Can you work these out from the model? Positions are in its coordinate system, mm. Face numbers are marked on the shaded views. A direction names the side the tool comes from. Coordinates: 2 decimals unless noted, no trailing zeros. Order: outer loops, then holes, each group sorted by start corner. A loop starts at its lowest first (then second) coordinate and runs counter-clockwise, first axis right, second up. Notation, with made-up numbers: (27, 82) -> (84, 82) arc R19 cw to (84, 87) -> close; hole circle Ø5 at (64, 70.25). An arc over 180 degrees is marked (long way). Return JSON: item names as keys, results as strings. Group by question number.
1) If we section it at A-A, the plane x = -5: Please give me the cut outline in (y, z), then the cut area to 3 significant figures.
2) For pin 1 (21.5 mm diameter, centred on x = -15.5, y = 22, fed in from -Z); pin 2 (4 mm diameter, centred on y = 12, z = 23, fed in from +X); pin 3 (4 mm diameter, centred on y = 12, z = 47, fed in from -X); pin 4 (12 mm diameter, centred on y = 44.5, z = 20.5, fed in from +X), each with a flat end and sliding along its axis, tell me the tip position at first contact or that it passes through.
3) If we section it at C-C, the plane y = 36: Please give me the cut outline in (x, z), then the cut area to 3 significant figures.
4) If we section it at D-D, the plane z = 47: Please give me the cut outline in (x, y).
5) If I drill on probe 1 along Y at (x, z) = (-44.15, 55); probe 2 along X at (y, z) = (58, 7); probe 3 along Z at (x, y) = (-28.5, 36), over which ranges is the centre line in solid material (lowest first)? Write a range as from..to.
6) For the marked faces 1 and 2, which set-ups out of +Z, -Z, +X, -X, +Y, -Y let a thin tool reach every point of the face, with its end or its side?
7) If we section it at B-B, the plane z = 56: Please give me the cut outline in (x, y), then the cut area to 3 significant figures.
8) Thinking about a two-plate mould opening in Z: for the marked faces 3, 4, 5 and 6, which applies, +Z half, -Z half, draft (parallel to the pull), parting line (faces both ways), or undercut?
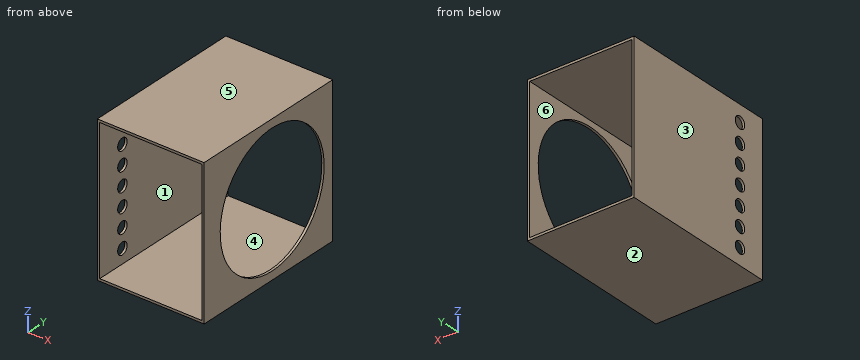
Autodesk Inventor part; units mm, degrees
ref_plane "YZ Plane" through (0, 0, 0) normal (1, 0, 0) x (0, 1, 0)
ref_plane "XZ Plane" through (0, 0, 0) normal (0, 1, 0) x (-1, 0, 0)
ref_plane "XY Plane" through (0, 0, 0) normal (0, 0, 1) x (1, 0, 0)
sketch "Boceto1" plane through (0, 0, 0) normal (0, 1, 0) x (-1, 0, 0)
  line L0 (0, 0) -> (45, 0)
  line L1 (45, 0) -> (45, 62)
  line L2 (45, 62) -> (0, 62)
  line L3 (0, 62) -> (0, 0)
  line L4 (44, 61) -> (1, 61)
  line L5 (1, 61) -> (1, 1)
  line L6 (1, 1) -> (44, 1)
  line L7 (44, 1) -> (44, 61)
  point P0 (22.5, 62)
  dimension "d0" = 1
  dimension "d1" = 1
  dimension "d2" = 1
  dimension "d3" = 1
  dimension "d4" = 43
  dimension "d5" = 60
extrude "Extrusión1" add sketch "Boceto1" along normal blind 68
sketch "Boceto2" plane through (0, 0, 62) normal (1, 0, 0) x (0, 0, -1)
  line L0 (0, 0) -> (62, 0)
  line L1 (62, 0) -> (62, 68)
  line L2 (0, 68) -> (62, 68)
  line L3 (0, 0) -> (0, 68)
  circle A0 centre (31, 36) radius 27.5
  point P0 (31, 68)
  dimension "d8" = 36
  dimension "d9" = 55
hole "Agujero1" at (0, 36, 31) direction (-1, 0, 0) diameter 55 depth 1
sketch "Boceto3" plane through (-45, 0, 0) normal (-1, 0, 0) x (0, 0, 1)
  line L0 (0, 0) -> (62, 0)
  line L1 (62, 0) -> (62, 68)
  line L2 (0, 68) -> (62, 68)
  line L3 (0, 0) -> (0, 68)
  circle A0 centre (31, 12) radius 2.5
  circle A1 centre (7, 12) radius 2.5
  circle A2 centre (55, 12) radius 2.5
  circle A3 centre (15, 12) radius 2.5
  circle A4 centre (23, 12) radius 2.5
  circle A5 centre (39, 12) radius 2.5
  circle A6 centre (47, 12) radius 2.5
  point P0 (0, 0)
  point P1 (31, 68)
  dimension "d17" = 5
  dimension "d18" = 12
  dimension "d19" = 5
  dimension "d20" = 5
  dimension "d21" = 24
  dimension "d22" = 48
  dimension "d24" = 3
  dimension "d25" = 3
  dimension "d26" = 3
  dimension "d27" = 3
  dimension "d28" = 3
hole "Agujero2" at (-45, 12, 7) at (-45, 12, 15) at (-45, 12, 23) at (-45, 12, 31) at (-45, 12, 39) at (-45, 12, 47) at (-45, 12, 55) direction (1, 0, 0) diameter 5 depth 1
properties part number "7-32" material "Latón, amarillo claro"
Result sheet:
{
 "1": {"outline": "(0, 0) -> (68, 0) -> (68, 1) -> (0, 1) -> close; (0, 61) -> (68, 61) -> (68, 62) -> (0, 62) -> close", "area": "136 mm2"},
 "2": {"pin 1": "stops at z = 0", "pin 2": "passes through", "pin 3": "stops at x = -1", "pin 4": "stops at x = -44"},
 "3": {"outline": "(-45, 0) -> (0, 0) -> (0, 3.5) -> (-1, 3.5) -> (-1, 1) -> (-44, 1) -> (-44, 61) -> (-1, 61) -> (-1, 58.5) -> (0, 58.5) -> (0, 62) -> (-45, 62) -> close", "area": "155 mm2"},
 "4": {"outline": "(-45, 0) -> (-44, 0) -> (-44, 9.5) -> (-45, 9.5) -> close; (-45, 14.5) -> (-44, 14.5) -> (-44, 68) -> (-45, 68) -> close; (-1, 0) -> (0, 0) -> (0, 13.63) -> (-1, 13.63) -> close; (-1, 58.37) -> (0, 58.37) -> (0, 68) -> (-1, 68) -> close"},
 "5": {"probe 1": "y = 0..9.5, 14.5..68", "probe 2": "x = -45..-44, -1..0", "probe 3": "z = 0..1, 61..62"},
 "6": {"face 1": "+Y, -Y", "face 2": "-Z, +X, -X, +Y, -Y"},
 "7": {"outline": "(-45, 0) -> (-44, 0) -> (-44, 9.71) -> (-45, 9.71) -> close; (-45, 14.29) -> (-44, 14.29) -> (-44, 68) -> (-45, 68) -> close; (-1, 0) -> (0, 0) -> (0, 24.54) -> (-1, 24.54) -> close; (-1, 47.46) -> (0, 47.46) -> (0, 68) -> (-1, 68) -> close", "area": "109 mm2"},
 "8": {"face 3": "draft", "face 4": "undercut", "face 5": "+Z half", "face 6": "undercut"}
}
